```python
from build123d import *

# Parameters (mm, degrees)
F1_DEPTH = 16.51
F3_DEPTH = 12.7
F5_DEPTH = 3.81


with BuildPart() as f1:
    # F0 (on Front) → F1 (new body)
    with BuildSketch(Plane.XZ):
        Polygon((-49.108937, 102.7169), (-131.373763, 102.7169), (-122.843154, 93.950309), (-96.143551, 93.950309), (-96.143551, 86.778201), (-117.512472, 86.778201), (-109.566309, 77.086523), (-96.143551, 77.086523), (-96.143551, 48.287213), (-78.310058, 63.821733), (-66.723436, 63.821733), (-55.69331, 74.407369), (-84.38962, 74.407369), (-84.38962, 93.950309), (-57.955489, 93.950309), align=None)
    extrude(amount=F1_DEPTH)

    # F2 (on face) → F3 (join)
    with BuildSketch(Plane.XZ.offset(16.51)):
        with BuildLine():
            ThreePointArc((-94.05135, 102.7169), (-90.24135, 106.5269), (-86.43135, 102.7169))
            Line((-86.43135, 102.7169), (-84.65335, 102.7169))
            ThreePointArc((-84.65335, 102.7169), (-90.24135, 108.3049), (-95.82935, 102.7169))
            Line((-95.82935, 102.7169), (-94.05135, 102.7169))
        make_face()
    extrude(amount=-F3_DEPTH)

    # F4 (on face) → F5 (cut)
    with BuildSketch(Plane.XZ.offset(16.51)):
        with BuildLine():
            Line((-86.43135, 102.7169), (-84.65335, 102.7169))
            ThreePointArc((-84.65335, 102.7169), (-90.24135, 108.3049), (-95.82935, 102.7169))
            Line((-95.82935, 102.7169), (-94.05135, 102.7169))
            ThreePointArc((-94.05135, 102.7169), (-90.24135, 106.5269), (-86.43135, 102.7169))
        make_face()
    extrude(amount=-F5_DEPTH, mode=Mode.SUBTRACT)


solid = f1.part
```
Part model, mm, in its own coordinate system. A direction names the side the tool comes from. Round coordinates to 2 decimals unless told otherwise and drop trailing zeros. Loops run counter-clockwise (first coordinate to the right, second up) from the corner with the lowest first, then second, coordinate; pieces in that order, holes last.
Item 1: Cut at D-D, the plane x = -116.5. Give the cut face in (y, z).
Item 2: Cut at B-B, the plane y = -6. Give the cut face in (x, z).
Item 3: 3-axis set-ups, long thin cutter, end or side, ignore diameter. For faces 1 (the face through (-107, -8, 86.778)), 2 (the face through (-90.325, -8.317, 106.526)), 3 (the face through (-53.594, -8.139, 98.272)), 4 (the face through (-96.144, -8, 63)): which of +Z, -Z, +X, -X, +Y, -Y reach the whole face in a straight line?
Item 4: Drill centre lines: line 1 (Z direction, x = -74, y = -1.5); line 2 (Z direction, x = -107.5, y = -6.25); line 3 (X direction, y = -8.5, z = 90). Where is each one in solid material? Low to high.
Item 5: Mould opens along Z. For faces 5 (the face through (-96.144, -8, 90)), 6 (the face through (-90, -16.51, 84)), 7 (the face through (-73, -8, 63.822)) say: +Z half, -Z half, draft (parallel to the pull), parting line (faces both ways), or undercut.
Item 6: Cut at A-A, the plane x = -72. Give the cut face in (y, z).
Item 7: Drop flat-ended pins along their axis: P1, Ø4.5, axis at x = -92.5, z = 105, coming from the -Y side; P2, Ø1, axis at x = -90.5, z = 61, coming from the +Y side; P3, Ø2, axis at x = -61, y = -10.5, coming from the +Z side; P4, Ø2, axis at y = -10.5, z = 75.5, coming from the -X side. Give the stop position or say it passes through.
Item 8: Cut at C-C, the plane y = -1.5. Give the cut face in (x, z).
A:
1. outline: (-16.51, 85.54) - (0, 85.54) - (0, 86.78) - (-16.51, 86.78) - close; (-16.51, 93.95) - (0, 93.95) - (0, 102.72) - (-16.51, 102.72) - close
2. outline: (-131.37, 102.72) - (-122.84, 93.95) - (-96.14, 93.95) - (-96.14, 86.78) - (-117.51, 86.78) - (-109.57, 77.09) - (-96.14, 77.09) - (-96.14, 48.29) - (-78.31, 63.82) - (-66.72, 63.82) - (-55.69, 74.41) - (-84.39, 74.41) - (-84.39, 93.95) - (-57.96, 93.95) - (-49.11, 102.72) - (-84.65, 102.72) arc R5.59 ccw to (-95.83, 102.72) - close; hole (-94.05, 102.72) - (-86.43, 102.72) arc R3.81 ccw to start
3. face 1: -X, +Y, -Y
3. face 2: +Y, -Y
3. face 3: +X, +Y, -Y
3. face 4: -Z, -X, +Y, -Y
4. line 1: z = 63.82 to 74.41, 93.95 to 102.72
4. line 2: z = 77.09 to 86.78, 93.95 to 102.72
4. line 3: x = -96.14 to -84.39
5. face 5: undercut
5. face 6: draft
5. face 7: -Z half
6. outline: (-16.51, 63.82) - (0, 63.82) - (0, 74.41) - (-16.51, 74.41) - close; (-16.51, 93.95) - (0, 93.95) - (0, 102.72) - (-16.51, 102.72) - close
7. P1: stops at y = -12.7
7. P2: stops at y = 0
7. P3: stops at z = 102.72
7. P4: stops at x = -96.14
8. outline: (-131.37, 102.72) - (-122.84, 93.95) - (-96.14, 93.95) - (-96.14, 86.78) - (-117.51, 86.78) - (-109.57, 77.09) - (-96.14, 77.09) - (-96.14, 48.29) - (-78.31, 63.82) - (-66.72, 63.82) - (-55.69, 74.41) - (-84.39, 74.41) - (-84.39, 93.95) - (-57.96, 93.95) - (-49.11, 102.72) - close
